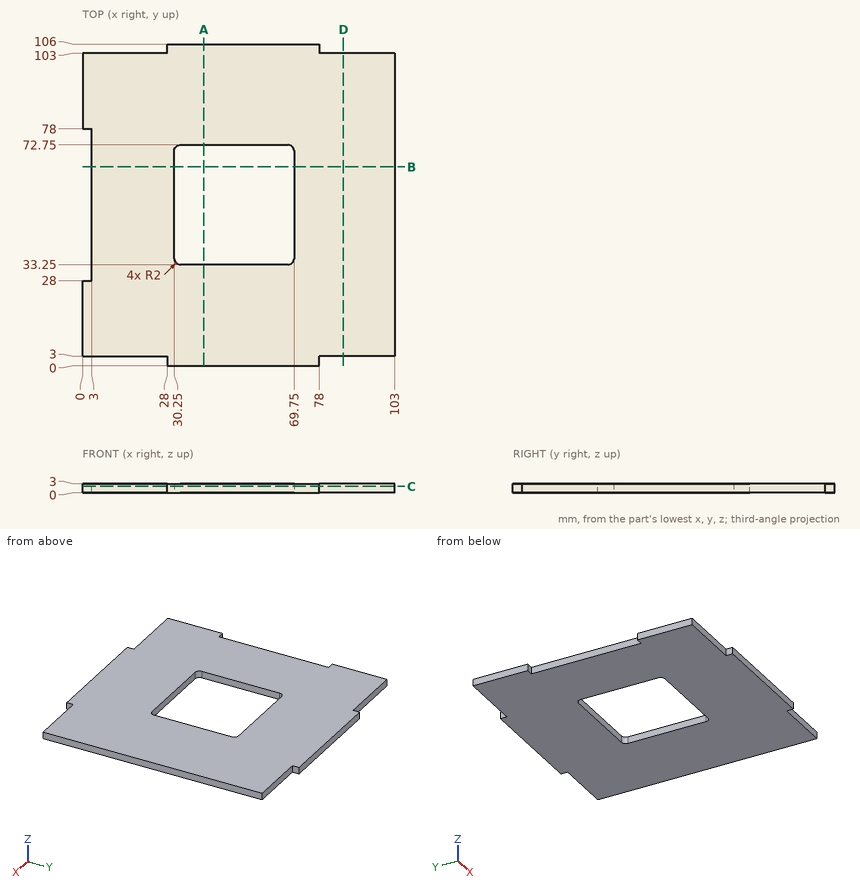
Source: three-view drawing plus pictorial views. Frame: mm from the lowest corner of the part. Round coordinates to 2 decimals unless told otherwise and drop trailing zeros. Loops run counter-clockwise (first coordinate to the right, second up) from the corner with the lowest first, then second, coordinate; pieces in that order, holes last. Notation, with made-up numbers: M 37.5,-14.5 L 82.5,-14.5 A31 ccw 82.5,17.5 Z; hole C -26,-32.75 d8. An arc over 180 degrees is marked long. Answer as CSV lines item,"result". Start each with the question number.
(1) Section B-B, the plane y = 65.5. Output: boundary loops of the cut face in (x, z).
(2) Section C-C, the plane z = 2.05. Output: boundary loops of the cut face in (x, y).
(3) Section A-A, the plane x = 40. Output: boundary loops of the cut face in (y, z).
(4) First-contact query: pin 1 (1.5 mm diameter, centred on y = 31.5, z = 2, fed in from -X); pin 2 (1.5 mm diameter, centred on x = 14.5, z = 2, fed in from -Y); pin 3 (0.9 mm diameter, centred on x = 91.5, z = 2, fed in from +Y); pin 4 (1.5 mm diameter, centred on x = 49, z = 1.5, fed in from -Y). Flat tips, straight axial feed; report the tip coordinate or a pass-through.
(5) Line query: line 1 (X direction, y = 49.5, z = 0.55); line 2 (Y direction, x = 50, z = 1.65); line 3 (Y direction, x = 85.5, z = 1.5). Output: solid intervals per line, ascending. Write a range as [from, to].
(6) Section D-D, the plane x = 86. Output: boundary loops of the cut face in (y, z).
Values found:
1,outline,"M 3,0 L 30.25,0 L 30.25,3 L 3,3 Z; M 69.75,0 L 103,0 L 103,3 L 69.75,3 Z"
2,outline,"M 0,3 L 28,3 L 28,0 L 78,0 L 78,3 L 103,3 L 103,103 L 78,103 L 78,106 L 28,106 L 28,103 L 0,103 L 0,78 L 3,78 L 3,28 L 0,28 Z; hole M 30.25,35.25 A2 ccw 32.25,33.25 L 67.75,33.25 A2 ccw 69.75,35.25 L 69.75,70.75 A2 ccw 67.75,72.75 L 32.25,72.75 A2 ccw 30.25,70.75 Z"
3,outline,"M 0,0 L 33.25,0 L 33.25,3 L 0,3 Z; M 72.75,0 L 106,0 L 106,3 L 72.75,3 Z"
4,pin 1,"stops at x = 3"
4,pin 2,"stops at y = 3"
4,pin 3,"stops at y = 103"
4,pin 4,"stops at y = 0"
5,line 1,"x = [3, 30.25], [69.75, 103]"
5,line 2,"y = [0, 33.25], [72.75, 106]"
5,line 3,"y = [3, 103]"
6,outline,"M 3,0 L 103,0 L 103,3 L 3,3 Z"
